```python
from build123d import *

# Parameters (mm, degrees)
SKETCH1_W           = 68
SKETCH1_H           = 35
BOSS_EXTRUDE1_DEPTH = 18
CUT_EXTRUDE1_DEPTH  = 5.28
SKETCH4_W           = 57.55
SKETCH4_H           = 1.8
BOSS_EXTRUDE2_DEPTH = 3.46
SKETCH5_R           = 2.5
CUT_EXTRUDE2_DEPTH  = 6
SKETCH6_W           = 35
SKETCH6_H           = 18
BOSS_EXTRUDE3_DEPTH = 16
CUT_EXTRUDE3_DEPTH  = 3
SKETCH9_W           = 80.3
SKETCH9_H           = 3.7
CUT_EXTRUDE4_DEPTH  = 20
SKETCH10_W          = 12
SKETCH10_H          = 8
CUT_EXTRUDE5_DEPTH  = 1
FILLET1_R           = 2
FILLET2_R           = 5


with BuildPart() as part:
    # Sketch1 → Boss-Extrude1 (new body)
    with BuildSketch(Plane(origin=(0, 0, 0), x_dir=(1, 0, 0), z_dir=(0, 1, 0))):
        Rectangle(SKETCH1_W, SKETCH1_H)
    extrude(amount=BOSS_EXTRUDE1_DEPTH)

    # Sketch3 → Cut-Extrude1 (cut)
    with BuildSketch(Plane.XZ):
        Polygon((31.7, -15.7), (31.7, 12.64), (-25.85, 12.64), (-25.85, 7.67), (-32.09, 7.67), (-32.09, -10.73), (-25.85, -10.73), (-25.85, -15.7), align=None)
    extrude(amount=-CUT_EXTRUDE1_DEPTH, mode=Mode.SUBTRACT)

    # Sketch4 → Boss-Extrude2 (add)
    with BuildSketch(Plane.XZ.offset(-5.28)):
        with Locations((2.925, 11.74)):
            Rectangle(SKETCH4_W, SKETCH4_H)
        with Locations((2.925, -14.8)):
            Rectangle(SKETCH4_W, SKETCH4_H)
    extrude(amount=BOSS_EXTRUDE2_DEPTH)

    # Sketch5 → Cut-Extrude2 (cut)
    with BuildSketch(Plane.XZ):
        with Locations(Location((29.5, 14.5, 0), (0, 0, 270))):
            Circle(SKETCH5_R)
        with Locations(Location((-30.5, -14, 0), (0, 0, 270))):
            Circle(SKETCH5_R)
    extrude(amount=-CUT_EXTRUDE2_DEPTH, mode=Mode.SUBTRACT)

    # Sketch6 → Boss-Extrude3 (add)
    with BuildSketch(Plane.ZY.offset(34)):
        with Locations((0, 9)):
            Rectangle(SKETCH6_W, SKETCH6_H)
    extrude(amount=BOSS_EXTRUDE3_DEPTH)

    # Sketch8 → Cut-Extrude3 (cut)
    with BuildSketch(Plane(origin=(34, 0, 0), x_dir=(0, 0, -1), z_dir=(1, 0, 0))):
        with BuildLine():
            Line((2.816168173, 4.079999973), (2.816168173, 2.879999987))
            ThreePointArc((2.816168173, 2.879999987), (3.167640032, 2.031471858), (4.016168161, 1.679999999))
            Line((4.016168161, 1.679999999), (10.956168078, 1.679999999))
            ThreePointArc((10.956168078, 1.679999999), (11.804696206, 2.031471858), (12.156168065, 2.879999987))
            Line((12.156168065, 2.879999987), (12.156168065, 4.079999973))
            ThreePointArc((12.156168065, 4.079999973), (11.804696206, 4.928528102), (10.956168078, 5.279999961))
            Line((10.956168078, 5.279999961), (4.016168161, 5.279999961))
            ThreePointArc((4.016168161, 5.279999961), (3.167640032, 4.928528102), (2.816168173, 4.079999973))
        make_face()
    extrude(amount=-CUT_EXTRUDE3_DEPTH, mode=Mode.SUBTRACT)

    # Sketch9 → Cut-Extrude4 (cut)
    with BuildSketch(Plane(origin=(0, 18, 0), x_dir=(1, 0, 0), z_dir=(0, 1, 0))):
        with Locations((-8, -3.4346612)):
            Rectangle(SKETCH9_W, SKETCH9_H)
    extrude(amount=-CUT_EXTRUDE4_DEPTH, mode=Mode.SUBTRACT)

    # Sketch10 → Cut-Extrude5 (cut)
    with BuildSketch(Plane(origin=(34, 0, 0), x_dir=(0, 0, -1), z_dir=(1, 0, 0))):
        with Locations((7.486168119, 3.47999998)):
            Rectangle(SKETCH10_W, SKETCH10_H)
    extrude(amount=-CUT_EXTRUDE5_DEPTH, mode=Mode.SUBTRACT)

    # Fillet1
    fillet1_edges = [part.edges().sort_by_distance(p)[0] for p in [
        (33.5, 7.47999998, -13.486168119),
        (33.5, 7.47999998, -1.486168119),
    ]]
    fillet(fillet1_edges, radius=FILLET1_R)

    # Fillet2
    fillet2_edges = [part.edges().sort_by_distance(p)[0] for p in [
        (-8, 18, 17.5),
        (-8, 18, -17.5),
    ]]
    fillet(fillet2_edges, radius=FILLET2_R)


solid = part.part
```
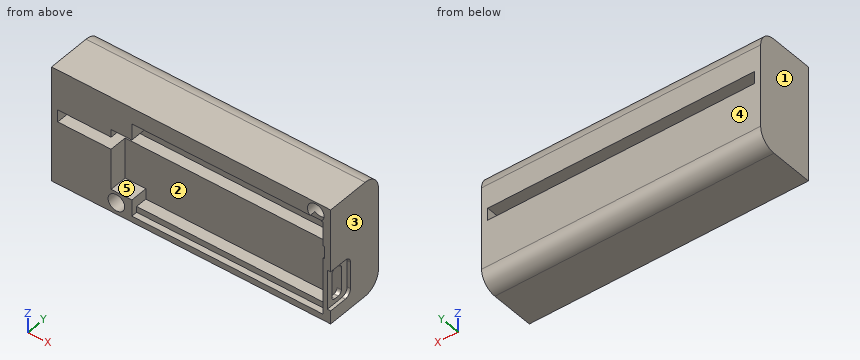
The listing builds one solid part. Answer for the finished solid, in the listing's coordinates (mm). Face numbers are marked on the shaded views. A direction names the side the tool comes from. Give positions to 0.01 mm unless a question says otherwise; leave off trailing zeros. Order: outer loops, then holes, each group sorted by start corner. A loop starts at its lowest first (then second) coordinate and runs counter-clockwise, first axis right, second up. Notation, with made-up numbers: (38, 15) -> (85, 15) arc R28 cw to (85, 33) -> close; hole circle Ø3 at (79, 55). An arc over 180 degrees is marked (long way). One line per item, written item: value.
1) Find the intervals of material crossed by line 1 (Z direction, x = -18, y = 4); line 2 (X direction, y = 1.65, z = -14); line 3 (X direction, y = 2.45, z = 14.5), in increasing order.
Reported:
line 1: z = -17.5 to -13.9, 10.84 to 17.5
line 2: x = -50 to -33, -28 to -25.85, 31.7 to 34
line 3: x = -50 to 27, 32 to 34
2) Flat-ended cylindrical pins translate along their axes: P1, Ø2, axis at x = -6.5, z = 8.5, coming from the -Y side; P2, Ø1.6, axis at y = 1.5, z = -7.5, coming from the +X side; P3, Ø0.8, axis at x = 33.5, z = -8.5, coming from the -Y side. Find the tip coordinate at first contact, or state that the pin passes through.
Reported:
P1: stops at y = 5.28
P2: stops at x = 33
P3: stops at y = 7.48
3) Determine the mould class of the marked faces 1, 2 and 3 for opening direction X: pulls with the +X half, pulls with the -X half, needs draft (parallel to the pull), parting line crosses it, or undercut.
Reported:
face 1: pulls with the -X half
face 2: undercut
face 3: pulls with the +X half
4) Find section A-A, the plane x = 3.5. Determine the outline of the cut face in (y, z).
Reported:
outline: (0, -17.5) -> (13, -17.5) arc R5 ccw to (18, -12.5) -> (18, 1.58) -> (5.28, 1.58) -> (5.28, -13.9) -> (1.82, -13.9) -> (1.82, -15.7) -> (0, -15.7) -> close; (0, 12.64) -> (1.82, 12.64) -> (1.82, 10.84) -> (5.28, 10.84) -> (5.28, 5.28) -> (18, 5.28) -> (18, 12.5) arc R5 ccw to (13, 17.5) -> (0, 17.5) -> close
5) A tool of negligible diameter and unlimited length cuts with its end or side. For the marked faces 4 and 5, from which of +Z, -Z, +X, -X, +Y, -Y can it reach the whole face along a straight path? Write none if from no direction.
Reported:
face 4: +Z, -Z, +X, -X, +Y
face 5: -Y
6) Find section C-C, the plane x = -30.5. Determine the outline of the cut face in (y, z), plus the area to 3 significant figures.
Reported:
outline: (0, -17.5) -> (13, -17.5) arc R5 ccw to (18, -12.5) -> (18, 1.58) -> (5.28, 1.58) -> (5.28, -10.73) -> (0, -10.73) -> (0, -11.5) -> (6, -11.5) -> (6, -16.5) -> (0, -16.5) -> close; (0, 7.67) -> (5.28, 7.67) -> (5.28, 5.28) -> (18, 5.28) -> (18, 12.5) arc R5 ccw to (13, 17.5) -> (0, 17.5) -> close
area: 445 mm^2
7) Find section D-D, the plane z = 9.5. Determine the outline of the cut face in (x, y), plus the area to 3 significant figures.
Reported:
outline: (-50, 0) -> (-25.85, 0) -> (-25.85, 5.28) -> (31.7, 5.28) -> (31.7, 0) -> (34, 0) -> (34, 18) -> (-50, 18) -> close
area: 1,210 mm^2
8) Find section B-B, the plane y = 12.25. Determine the outline of the cut face in (x, z), plus the area to 3 significant figures.
Reported:
outline: (-50, -17.5) -> (34, -17.5) -> (34, 17.5) -> (-50, 17.5) -> close; hole (-48.15, 1.58) -> (32.15, 1.58) -> (32.15, 5.28) -> (-48.15, 5.28) -> close
area: 2,640 mm^2
